Could you check a few things on this drawing? It's one solid part, dimensions in mm from its lowest x, y, z. Give positions to 0.01 mm unless a question says otherwise; leave off trailing zeros. Order: outer loops, then holes, each group sorted by start corner. A loop starts at its lowest first (then second) coordinate and runs counter-clockwise, first axis right, second up. Notation, with made-up numbers: (-24.75, 21.5) - (3.25, 21.5) arc R17 ccw to (3.25, 27.5) - close; hole circle Ø6 at (53, 25). An arc over 180 degrees is marked (long way). Put each result on its own line as item: value.
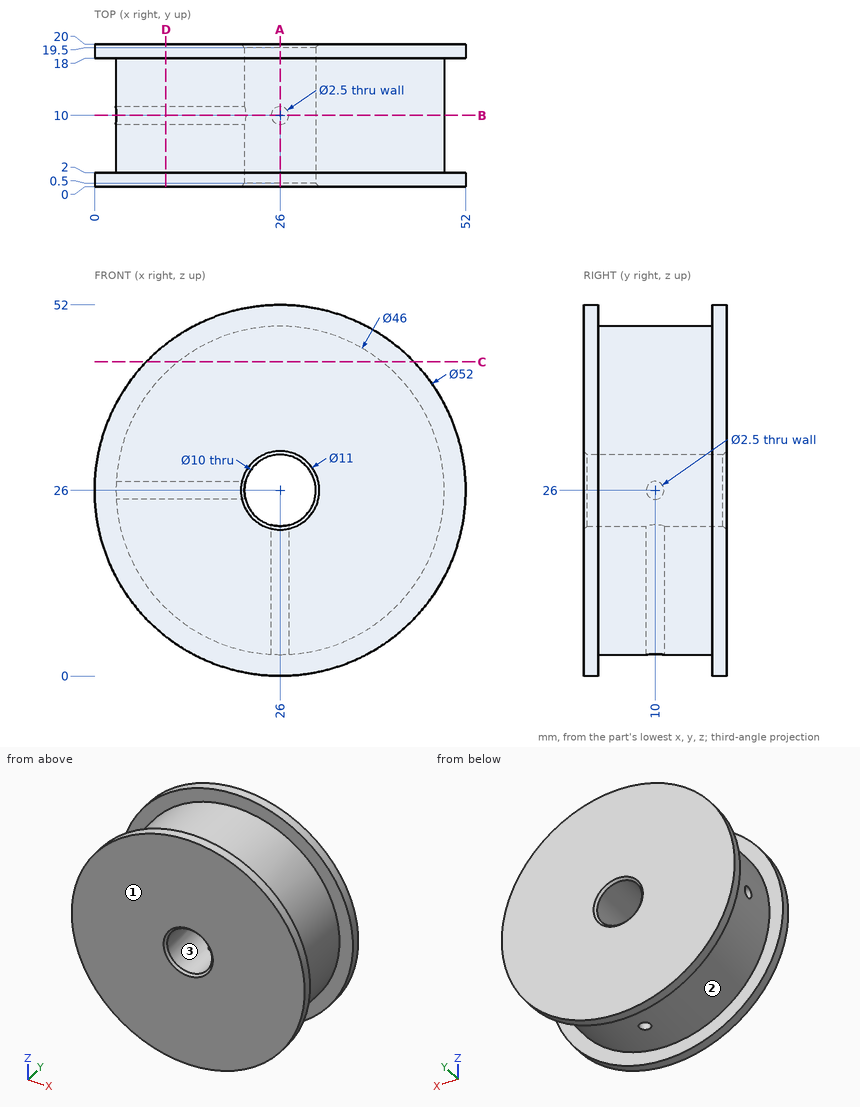
1) I'm going to push flat-ended pins straight in: pin 1 (1 mm diameter, centred on x = 17, z = 10.5, fed in from -Y); pin 2 (1.5 mm diameter, centred on x = 24, y = 3, fed in from -Z); pin 3 (2 mm diameter, centred on y = 10, z = 26, fed in from -X); pin 4 (8 mm diameter, centred on y = 14.5, z = 7.5, fed in from -X). Where does each tip first touch, or does it pass through?
Filled in:
pin 1: stops at y = 0
pin 2: stops at z = 3.03
pin 3: stops at x = 30.9
pin 4: stops at x = 5.96
2) Suppose I cut it at A-A, the plane x = 26. List the corners of the cut face in (y, z) for me.
Filled in:
outline: (0, 0) - (2, 0) - (2, 3) - (8.75, 3) - (8.75, 21) - (0.5, 21) - (0, 20.5) - close; (0, 31.5) - (0.5, 31) - (19.5, 31) - (20, 31.5) - (20, 52) - (18, 52) - (18, 49) - (2, 49) - (2, 52) - (0, 52) - close; (11.25, 3) - (18, 3) - (18, 0) - (20, 0) - (20, 20.5) - (19.5, 21) - (11.25, 21) - close
3) We'd pull the mould along X, two halves only. Please class the marked faces 1, 2 and 3: pulls with the +X half, pulls with the -X half, needs draft (parallel to the pull), parting line crosses it, or undercut.
Filled in:
face 1: needs draft
face 2: parting line crosses it
face 3: undercut
4) If I drill on line 1 (Y direction, x = 26, z = 8); line 2 (X direction, y = 15, z = 26); line 3 (Z direction, x = 17, y = 10), over which ranges is the centre line in solid material (lowest first)? Write a range as [from, to].
Filled in:
line 1: y = [0, 8.75], [11.25, 20]
line 2: x = [3, 21], [31, 49]
line 3: z = [4.83, 24.75], [27.25, 47.17]
5) Suppose I cut it at D-D, the plane x = 10. List the corners of the cut face in (y, z) for me, and give its area (3 significant figures).
Filled in:
outline: (0, 5.51) - (2, 5.51) - (2, 9.48) - (18, 9.48) - (18, 5.51) - (20, 5.51) - (20, 46.49) - (18, 46.49) - (18, 42.52) - (2, 42.52) - (2, 46.49) - (0, 46.49) - close; hole circle Ø2.5 at (10, 26)
area: 688 mm^2
6) Suppose I cut it at C-C, the plane z = 44. List the corners of the cut face in (x, y) for me.
Filled in:
outline: (7.24, 0) - (44.76, 0) - (44.76, 2) - (40.32, 2) - (40.32, 18) - (44.76, 18) - (44.76, 20) - (7.24, 20) - (7.24, 18) - (11.68, 18) - (11.68, 2) - (7.24, 2) - close
7) Suppose I cut it at B-B, the plane y = 10. List the corners of the cut face in (x, z) for me, and give its area (3 significant figures).
Filled in:
outline: (3.03, 24.75) arc R23 ccw to (24.75, 3.03) - (24.75, 21.16) arc R5 cw to (21.16, 24.75) - close; (3.03, 27.25) - (21.16, 27.25) arc R5 cw (long way) to (27.25, 21.16) - (27.25, 3.03) arc R23 ccw (long way) to start
area: 1,490 mm^2
